Here's the drawing with two shaded views (mm, measured from the low corner). I have some questions. Round coordinates to 2 decimals unless told otherwise and drop trailing zeros. Write each loop counter-clockwise with the first axis right and the second up, starting at its lowest first coordinate (ties: lowest second). Pieces come first, ordered by that corner, then holes.
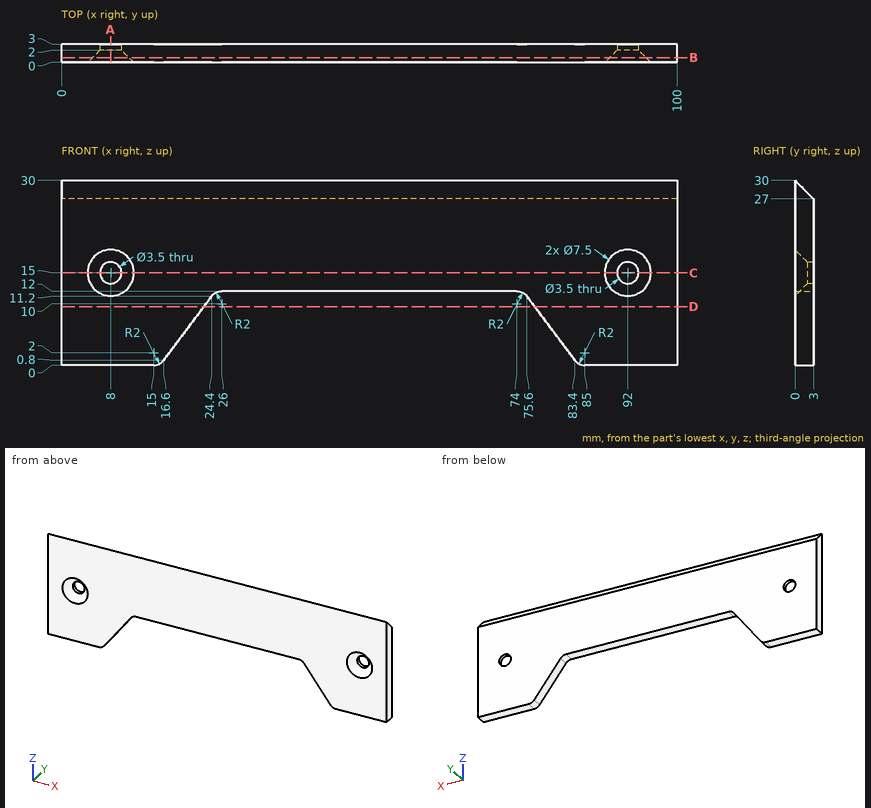
Q1. Imagine slicing it at C-C, the plane z = 15. Write out the boundary of the cut face in (x, y), then the cut area to 3 significant figures.
Q2. I'm going to push flat-ended pins straight in: pin 1 Ø1 at (y, z) = (1, 14.5) entering from -X; pin 2 Ø0.9 at (x, y) = (53, 1) entering from -Z. Where does each tip first touch, or does it pass through?
Q3. Imagine slicing it at D-D, the plane z = 9.5. Write out the boundary of the cut face in (x, y) (3 decimals), then the cut area to 3 significant figures.
Q4. Imagine slicing it at B-B, the plane y = 0.8. Write out the boundary of the cut face in (x, z), then the cut area to 3 significant figures.
Q5. If I drill on L1, parallel to X at y = 0.4, z = 13.5; L2, parallel to X at y = 1.95, z = 15.25; L3, parallel to Z at x = 8, y = 2.2, over which ranges is the centre line in solid material (lowest first)?
Q6. Imagine slicing it at A-A, the plane x = 8. Write out the boundary of the cut face in (y, z), then the cut area to 3 significant figures.
Results found:
1. outline: (0, 0) - (4.25, 0) - (6.25, 2) - (6.25, 3) - (0, 3) - close; (9.75, 2) - (11.75, 0) - (88.25, 0) - (90.25, 2) - (90.25, 3) - (9.75, 3) - close; (93.75, 2) - (95.75, 0) - (100, 0) - (100, 3) - (93.75, 3) - close
1. area: 271 mm2
2. pin 1: stops at x = 0
2. pin 2: stops at z = 12
3. outline: (0, 0) - (23.125, 0) - (23.125, 3) - (0, 3) - close; (76.875, 0) - (100, 0) - (100, 3) - (76.875, 3) - close
3. area: 139 mm2
4. outline: (0, 0) - (15, 0) arc R2 ccw to (16.6, 0.8) - (24.4, 11.2) arc R2 cw to (26, 12) - (74, 12) arc R2 cw to (75.6, 11.2) - (83.4, 0.8) arc R2 ccw to (85, 0) - (100, 0) - (100, 29.2) - (0, 29.2) - close; hole circle Ø5.9 at (8, 15); hole circle Ø5.9 at (92, 15)
4. area: 2,160 mm2
5. L1: x = 0 to 5, 11 to 89, 95 to 100
5. L2: x = 0 to 6.22, 9.78 to 90.22, 93.78 to 100
5. L3: z = 0 to 13.25, 16.75 to 27.8
6. outline: (0, 0) - (3, 0) - (3, 13.25) - (2, 13.25) - (0, 11.25) - close; (0, 18.75) - (2, 16.75) - (3, 16.75) - (3, 27) - (0, 30) - close
6. area: 71.0 mm2
